from build123d import *

# Parameters (mm, degrees)
SKETCH3_R               = 8
BOSS_EXTRUDE1_DEPTH     = 48.633157895
CUT_EXTRUDE1_DEPTH      = 13.989776257
CUT_EXTRUDE1_DEPTH_BACK = 13.989776257
BOSS_EXTRUDE2_DEPTH     = 1.2
CUT_EXTRUDE2_DEPTH      = 1.6
SKETCH8_R               = 1.4
SKETCH8_R_2             = 1.6
CUT_EXTRUDE3_DEPTH      = 2.64160469
CUT_EXTRUDE3_DEPTH_BACK = 52.97615102
CUT_EXTRUDE4_DEPTH      = 52.97615102


with BuildPart() as part:
    # Sketch3 → Boss-Extrude1 (new body)
    with BuildSketch(Plane(origin=(-20.344467381, 196.178792599, 0), x_dir=(-0.994665758, -0.103150523, 0), z_dir=(0.103150523, -0.994665758, 0))):
        with Locations((-10.431405186, 0)):
            Circle(SKETCH3_R)
    extrude(amount=BOSS_EXTRUDE1_DEPTH)

    # Sketch4 → Cut-Extrude1 (cut, two sides)
    with BuildSketch(Plane(origin=(10.375761543, 1.076004901, 0), x_dir=(0.103150523, -0.994665758, 0), z_dir=(-0.994665758, -0.103150523, 0))) as cut_extrude1_sk:
        Polygon((-197.230869842, 0), (-189.230869842, 8), (-197.230869842, 8), align=None)
        Polygon((-156.597711947, 8), (-148.597711947, 8), (-148.597711947, 0), align=None)
    extrude(amount=CUT_EXTRUDE1_DEPTH, mode=Mode.SUBTRACT)
    extrude(cut_extrude1_sk.sketch, amount=-CUT_EXTRUDE1_DEPTH_BACK, mode=Mode.SUBTRACT)

    # Sketch5 → Boss-Extrude2 (add, symmetric)
    with BuildSketch(Plane(origin=(10.375761543, 1.076004901, 0), x_dir=(0.103150523, -0.994665758, 0), z_dir=(-0.994665758, -0.103150523, 0))):
        with BuildLine():
            Line((-148.597711947, -2.8), (-146.172840817, 1.4))
            ThreePointArc((-146.172840817, 1.4), (-148.232238609, 2.776045612), (-150.577610935, 1.979898987))
            Line((-150.577610935, 1.979898987), (-148.597711947, 0))
            Line((-148.597711947, 0), (-148.597711947, -2.8))
        make_face()
    extrude(amount=BOSS_EXTRUDE2_DEPTH, both=True)

    # Sketch7 → Cut-Extrude2 (cut, symmetric)
    with BuildSketch(Plane(origin=(10.375761543, 1.076004901, 0), x_dir=(0.103150523, -0.994665758, 0), z_dir=(-0.994665758, -0.103150523, 0))):
        with BuildLine():
            Line((-194.968128142, 2.2627417), (-197.230869842, 0))
            Line((-197.230869842, 0), (-197.230869842, -3.2))
            ThreePointArc((-197.230869842, -3.2), (-194.274455338, -1.224586984), (-194.968128142, 2.2627417))
        make_face()
    extrude(amount=CUT_EXTRUDE2_DEPTH, both=True, mode=Mode.SUBTRACT)

    # Sketch8 → Cut-Extrude3 (cut, two sides)
    with BuildSketch(Plane(origin=(-20.344467381, 196.178792599, 0), x_dir=(0.994665758, 0.103150523, 0), z_dir=(-0.103150523, 0.994665758, 0))) as cut_extrude3_sk:
        with Locations((10.431405186, -5.5)):
            Circle(SKETCH8_R)
        with Locations((6.831405186, 3)):
            Circle(SKETCH8_R_2)
        with Locations((14.031405186, 3)):
            Circle(SKETCH8_R_2)
    extrude(amount=CUT_EXTRUDE3_DEPTH, mode=Mode.SUBTRACT)
    extrude(cut_extrude3_sk.sketch, amount=-CUT_EXTRUDE3_DEPTH_BACK, mode=Mode.SUBTRACT)

    # Sketch9 → Cut-Extrude4 (cut, through all)
    with BuildSketch(Plane(origin=(-20.344467381, 196.178792599, 0), x_dir=(0.994665758, 0.103150523, 0), z_dir=(-0.103150523, 0.994665758, 0))):
        with BuildLine():
            Line((7.933405986, 7.6), (12.929404385, 7.6))
            ThreePointArc((12.929404385, 7.6), (10.431405186, 8), (7.933405986, 7.6))
        make_face()
        with BuildLine():
            Line((7.933405986, -7.6), (12.929404385, -7.6))
            ThreePointArc((12.929404385, -7.6), (10.431405186, -8), (7.933405986, -7.6))
        make_face()
    extrude(amount=-CUT_EXTRUDE4_DEPTH, mode=Mode.SUBTRACT)


solid = part.part
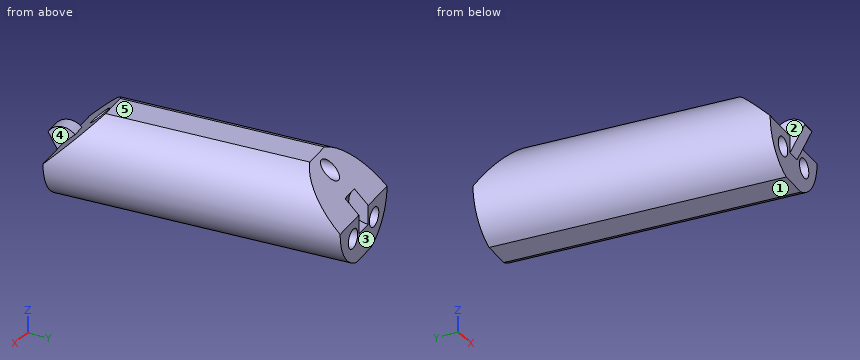
Source: CAD feature listing. Evaluate the final solid. Frame: model axes, mm. Face numbers are marked on the shaded views. A direction names the side the tool comes from. Coordinates: 2 decimals unless noted, no trailing zeros. Write each loop counter-clockwise with the first axis right and the second up, starting at its lowest first coordinate (ties: lowest second). Pieces come first, ordered by that corner, then holes. Notation, with made-up numbers: M -11.5,14 L 42.5,14 A16 cw 42.5,23 Z; hole C 79,49.25 d3. An arc over 180 degrees is marked long. Use a Markdown table: item, result.
1) Section C-C, the plane y = 176. Give the number of separate pieces and of enclosed holes in the cut face, then the cut area to 3 significant figures.
Conclusion:
| item | result |
|---|---|
| separate pieces | 1 |
| enclosed holes | 3 |
| area | 177 mm^2 |
2) Reachability of the marked faces 4 and 5 from +Z, -Z, +X, -X, +Y, -Y: full face, straight path, thin tool, end or side. Return the list, or none.
Conclusion:
| item | result |
|---|---|
| face 4 | +Z, +X |
| face 5 | +Z, +X, -X, +Y, -Y |
3) First-contact query: pin 1 Ø1 at (x, y) = (-0.5, 167.5) entering from -Z; pin 2 Ø6 at (y, z) = (175.5, 1.5) entering from +X; pin 3 Ø3 at (x, z) = (-6, -2.5) entering from +Y. Flat tips, straight axial feed; report the tip coordinate or a pass-through.
Conclusion:
| item | result |
|---|---|
| pin 1 | stops at z = -5.46 |
| pin 2 | stops at x = 0.61 |
| pin 3 | stops at y = 197.82 |
4) Mould query, pull axis X, two halves, no side actions, for the marked faces 1, 2 and 3. Classes: pulls with the +X half, pulls with the -X half, needs draft (parallel to the pull), parting line crosses it, or undercut.
Conclusion:
| item | result |
|---|---|
| face 1 | needs draft |
| face 2 | undercut |
| face 3 | pulls with the -X half |
5) Section A-A, the plane z = -4. Output: boundary loops of the cut face in (x, y), then the cut area to 3 significant figures.
Conclusion:
| item | result |
|---|---|
| outline | M -16.86,196.54 L -11.84,148.17 L -9.78,148.38 L -14.79,196.75 Z; M -12.31,197.01 L -7.29,148.64 L -2.61,149.12 L -7.63,197.5 Z; M -5.15,197.75 L -0.13,149.38 L 1.94,149.6 L -3.08,197.97 Z |
| area | 431 mm^2 |
6) Section B-B, the plane z = -0.5. Output: boundary loops of the cut face in (x, y).
Conclusion:
| item | result |
|---|---|
| outline | M -17.91,196.43 L -12.89,148.06 L -6.15,148.76 L -6.01,147.44 L -3.62,147.68 L -3.76,149 L 2.99,149.7 L -2.03,198.08 L -8.38,197.42 L -8.05,194.28 L -11.23,193.95 L -11.56,197.09 Z |
7) Ray query, L1, parallel to X at y = 187.5, z = -2; L2, parallel to X at y = 182, z = -3.75; L3, parallel to X at y = 158.5, z = 6.5. Return the intervals inside material, ascending.
Conclusion:
| item | result |
|---|---|
| L1 | x = -16.74 to -13.83, -11.32 to -6.59, -4.08 to -1.17 |
| L2 | x = -15.49 to -13.43, -10.59 to -6.19, -3.35 to -1.28 |
| L3 | x = -10.64 to -6.93, -4.96 to -1.26 |
